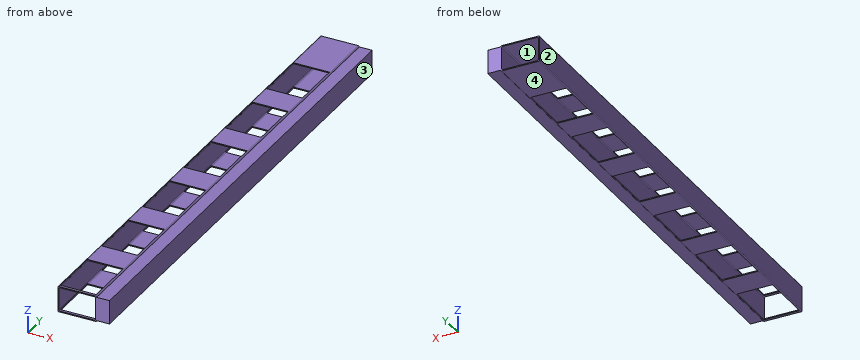
```python
from build123d import *

# Parameters (mm, degrees)
F0_W     = 75
F0_H     = 50
F0_W_2   = 71
F0_H_2   = 46
F1_DEPTH = 970
F3_R     = 2
F4_R     = 2
F2_W     = 69
F2_H     = 100
F5_DEPTH = 60
F6_DEPTH = 25


with BuildPart() as f1:
    # F0 (on Front) → F1 (new body)
    with BuildSketch(Plane.XZ):
        Rectangle(F0_W, F0_H)
        Rectangle(F0_W_2, F0_H_2, mode=Mode.SUBTRACT)
    extrude(amount=F1_DEPTH)

    # F3
    f3_edges = [f1.edges().sort_by_distance(p)[0] for p in [
        (-37.5, -485, 25),
        (37.5, -485, 25),
        (37.5, -485, -25),
        (-37.5, -485, -25),
    ]]
    fillet(f3_edges, radius=F3_R)

    # F4
    f4_edges = [f1.edges().sort_by_distance(p)[0] for p in [
        (-35.5, -485, 23),
        (-35.5, -485, -23),
        (35.5, -485, -23),
        (35.5, -485, 23),
    ]]
    fillet(f4_edges, radius=F4_R)

    # F2 (on face) → F5 (cut)
    with BuildSketch(Plane.XY.offset(25)):
        with Locations((-0.4652442876, -915)):
            Rectangle(F2_W, F2_H)
        with Locations((-0.4652442876, -762.69)):
            Rectangle(F2_W, F2_H)
        with Locations((-0.4652442876, -610.38)):
            Rectangle(F2_W, F2_H)
        with Locations((-0.4652442876, -458.07)):
            Rectangle(F2_W, F2_H)
        with Locations((-0.4652442876, -305.76)):
            Rectangle(F2_W, F2_H)
        with Locations((-0.4652442876, -153.45)):
            Rectangle(F2_W, F2_H)
    extrude(amount=-F5_DEPTH, mode=Mode.SUBTRACT)

    # F6 (add): a face of the model
    f6_faces = [f1.faces().sort_by_distance(p)[0] for p in [
        (37.5, -485, 0),
    ]]
    extrude(f6_faces, amount=F6_DEPTH)


solid = f1.part
```
Geometry check sheet. Reference: the model listing, model coordinates, mm. Face numbers are marked on the shaded views. Round coordinates to 2 decimals unless told otherwise and drop trailing zeros. Order: outer loops, then holes, each group sorted by start corner. A loop starts at its lowest first (then second) coordinate and runs counter-clockwise, first axis right, second up. Notation, with made-up numbers: (-35, -16.75) - (16, -16.75) arc R6 cw to (16, -7.75) - close; hole circle Ø9 at (-24, 59). An arc over 180 degrees is marked (long way). Use a Markdown table: item, result. Add a question column.
1) Gauge pin test, flat end, axial feed: P1, Ø2.5, axis at y = -452, z = -24.5, coming from the -X side. Record the tip position at first contact, or that the pin passes through.
2) Section check C-C (x = -2). Count the separate pieces of the cut face and the enclosed holes in it, then the cut area to 3 significant figures.
3) Section check B-B (y = -418.5). Record the cut outline in (x, z).
4) Mould release check, pull along X, two halves, no side actions. Record for the marked faces 1, 2, 3 and 4: released by +X, released by -X, zero draft, split by the parting line, or undercut.
5) Section check D-D (x = 45.5). Record the cut outline in (y, z).
6) Thickness scan on line 1 along X through (y, z) = (-324, -1); line 2 along Z through (x, y) = (11, -696.5); line 3 along Z through (x, y) = (51, -395). Record the ranges inside material, lowest first.
7) Section check A-A (z = 9). Record the cut outline in (x, y), then the cut area to 3 significant figures.
Established:
| question | item | result |
|---|---|---|
| 1 | P1 | x = -37.48 |
| 2 | separate pieces | 14 |
| 2 | enclosed holes | 0 |
| 2 | area | 1,480 mm2 |
| 3 | outline | (-37.5, -23) arc R2 ccw to (-35.5, -25) - (-34.97, -25) - (-34.97, -22.36) arc R2 cw to (-35.5, -21) - (-35.5, 21) arc R2 cw to (-34.97, 22.36) - (-34.97, 25) - (-35.5, 25) arc R2 ccw to (-37.5, 23) - close; (34.03, -25) - (35.5, -25) arc R2 ccw to (37.5, -23) - (62.5, -23) - (62.5, 23) - (37.5, 23) arc R2 ccw to (35.5, 25) - (34.03, 25) - (34.03, 22.93) arc R2 cw to (35.5, 21) - (35.5, -21) arc R2 cw to (34.03, -22.93) - close |
| 4 | face 1 | undercut |
| 4 | face 2 | released by -X |
| 4 | face 3 | released by +X |
| 4 | face 4 | zero draft |
| 5 | outline | (-970, -23) - (0, -23) - (0, 23) - (-970, 23) - close |
| 6 | line 1 | -37.5 to -35.5, 35.5 to 62.5 |
| 6 | line 2 | -25 to -23, 23 to 25 |
| 6 | line 3 | -23 to 23 |
| 7 | outline | (-37.5, -970) - (-35.5, -970) - (-35.5, 0) - (-37.5, 0) - close; (35.5, -970) - (62.5, -970) - (62.5, 0) - (35.5, 0) - close |
| 7 | area | 28,100 mm2 |
